```python
from build123d import *

# Parameters (mm, degrees)
F0_R     = 1.625
F0_R_2   = 2.5
F1_DEPTH = 1


with BuildPart() as f1:
    # F0 (on Top) → F1 (new body)
    with BuildSketch(Plane.XY):
        with BuildLine():
            ThreePointArc((3, 9.5), (0, 12.5), (-3, 9.5))
            Line((-3, 9.5), (-3, 6))
            ThreePointArc((-3, 6), (-3.87868, 3.87868), (-6, 3))
            Line((-6, 3), (-8, 3))
            ThreePointArc((-8, 3), (-11, 0), (-8, -3))
            Line((-8, -3), (-6, -3))
            ThreePointArc((-6, -3), (-3.87868, -3.87868), (-3, -6))
            Line((-3, -6), (-3, -9.5))
            ThreePointArc((-3, -9.5), (0, -12.5), (3, -9.5))
            Line((3, -9.5), (3, -6))
            ThreePointArc((3, -6), (3.87868, -3.87868), (6, -3))
            Line((6, -3), (8, -3))
            ThreePointArc((8, -3), (11, 0), (8, 3))
            Line((8, 3), (6, 3))
            ThreePointArc((6, 3), (3.87868, 3.87868), (3, 6))
            Line((3, 6), (3, 9.5))
        make_face()
        with Locations((0, -9.5)):
            Circle(F0_R, mode=Mode.SUBTRACT)
        with Locations((-8, 0)):
            Circle(F0_R, mode=Mode.SUBTRACT)
        Circle(F0_R_2, mode=Mode.SUBTRACT)
        with Locations((8, 0)):
            Circle(F0_R, mode=Mode.SUBTRACT)
        with Locations((0, 9.5)):
            Circle(F0_R, mode=Mode.SUBTRACT)
    extrude(amount=F1_DEPTH)


solid = f1.part
```
Part model, mm, in its own coordinate system. A direction names the side the tool comes from. Coordinates: 2 decimals unless noted, no trailing zeros. Order: outer loops, then holes, each group sorted by start corner. A loop starts at its lowest first (then second) coordinate and runs counter-clockwise, first axis right, second up. Notation, with made-up numbers: (-5.5, -34) - (18.5, -34) arc R4 ccw to (18.5, -29) - close; hole circle Ø7 at (70, -38). An arc over 180 degrees is marked (long way). Return JSON: item names as keys, results as strings. Group by question number.
Item 1: Pin check, flat tips, straight feed: pin 1 (0.5 mm diameter, centred on y = 8, z = 0.5, fed in from +X); pin 2 (0.5 mm diameter, centred on x = 7.5, z = 0.5, fed in from +Y). Stop position of each tip, or through.
Item 2: Drill centre lines: probe 1 along Y at (x, z) = (0, 0.65) (3 decimals); probe 2 along Y at (x, z) = (-8, 0.65) (3 decimals); probe 3 along X at (y, z) = (-7.75, 0.6). Where is each one in solid material? Low to high. Write a range as from..to.
Item 3: Cut at C-C (z = 0.7). List the corners of the cut face in (x, y) (3 decimals).
Item 4: Pull direction Y, two halves, no side cores. Call faces 4 (the face through (-3.86, 3.9, 0.49)), 5 (the face through (11, -0.1, 0.5)), 6 (the face through (9.55, 0.49, 0.49)): pulls with the +Y half, pulls with the -Y half, needs draft (parallel to the pull), parting line crosses it, or undercut.
Item 5: Which spindle directions (+Z, -Z, +X, -X, +Y, -Y) get a long thin tool onto all of the face, cutting with end or side? Do faces 1 (the face through (7, -3, 0.5)), 2 (the face through (-3, 7.8, 0.5)), 3 (the face through (7, 3, 0.5)). Say none if no direction does.
Item 6: Cut at A-A (x = 0). List the corners of the cut face in (y, z) (3 decimals).
Item 7: Cut at D-D (y = 9). List the corners of the cut face in (x, z), plus the area to 3 significant figures.
Item 8: Cut at B-B (y = 0). List the corners of the cut face in (x, z) (3 decimals), plus the area to 3 significant figures.
Check values:
{
 "1": {"pin 1": "stops at x = 3", "pin 2": "stops at y = 3"},
 "2": {"probe 1": "y = -12.5..-11.125, -7.875..-2.5, 2.5..7.875, 11.125..12.5", "probe 2": "y = -3..-1.625, 1.625..3", "probe 3": "x = -3..3"},
 "3": {"outline": "(-8, -3) - (-6, -3) arc R3 cw to (-3, -6) - (-3, -9.5) arc R3 ccw to (3, -9.5) - (3, -6) arc R3 cw to (6, -3) - (8, -3) arc R3 ccw to (8, 3) - (6, 3) arc R3 cw to (3, 6) - (3, 9.5) arc R3 ccw to (-3, 9.5) - (-3, 6) arc R3 cw to (-6, 3) - (-8, 3) arc R3 ccw to start; hole circle Ø3.25 at (-8, 0); hole circle Ø5 at (0, 0); hole circle Ø3.25 at (0, -9.5); hole circle Ø3.25 at (0, 9.5); hole circle Ø3.25 at (8, 0)"},
 "4": {"face 4": "pulls with the +Y half", "face 5": "parting line crosses it", "face 6": "undercut"},
 "5": {"face 1": "+Z, -Z, +X, -Y", "face 2": "+Z, -Z, -X, +Y", "face 3": "+Z, -Z, +X, +Y"},
 "6": {"outline": "(-12.5, 0) - (-11.125, 0) - (-11.125, 1) - (-12.5, 1) - close; (-7.875, 0) - (-2.5, 0) - (-2.5, 1) - (-7.875, 1) - close; (2.5, 0) - (7.875, 0) - (7.875, 1) - (2.5, 1) - close; (11.125, 0) - (12.5, 0) - (12.5, 1) - (11.125, 1) - close"},
 "7": {"outline": "(-3, 0) - (-1.55, 0) - (-1.55, 1) - (-3, 1) - close; (1.55, 0) - (3, 0) - (3, 1) - (1.55, 1) - close", "area": "2.91 mm2"},
 "8": {"outline": "(-11, 0) - (-9.625, 0) - (-9.625, 1) - (-11, 1) - close; (-6.375, 0) - (-2.5, 0) - (-2.5, 1) - (-6.375, 1) - close; (2.5, 0) - (6.375, 0) - (6.375, 1) - (2.5, 1) - close; (9.625, 0) - (11, 0) - (11, 1) - (9.625, 1) - close", "area": "10.5 mm2"}
}
